The model under review builds one solid part; all positions refer to its coordinate system, in mm. A direction names the side the tool comes from. Coordinates: 2 decimals unless noted, no trailing zeros. Loops run counter-clockwise (first coordinate to the right, second up) from the corner with the lowest first, then second, coordinate; pieces in that order, holes last. Notation, with made-up numbers: (-23.5, 41) - (27.5, 41) arc R7 cw to (27.5, 54) - close; hole circle Ø5 at (50.25, -15.5). An arc over 180 degrees is marked (long way). Answer in a Markdown table with one row per item. Add a question column.
(1) We need section C-C on z = 113.5. Write out the cut boundary in (x, y).
(2) We need section D-D on y = 113. Write out the cut boundary in (x, z).
(3) Mouldability with a two-part tool opening along X and no side actions: class faces 3 (the cylindrical face through (95.38, 30.04, 152.97)), 4 (the flat face through (-95, -29, 310)), 5 (the cylindrical face through (52.684, 82.634, 152.83)) as +X half, -X half, draft (parallel to the pull), parting line (faces both ways), or undercut.
(4) We need section A-A on y = 0. Write out the cut boundary in (x, z).
(5) For P1, Ø4, axis at y = -37, z = 194, coming from the +X side (3 decimals); P2, Ø2, axis at y = 28.5, z = 68, coming from the +X side; P3, Ø5, axis at y = 25.5, z = 44.5, coming from the +X side, all flat-tipped, find the tip position at first contact; note any pin that passes through.
(6) Machinability: for faces 1 (the flat face through (-95, -29, 0)), 2 (the flat face through (-95, 33, 10)), which of the approach directions +Z, -Z, +X, -X, +Y, -Y give a long, thin tool a straight path to every point of the face, cutting with its end or side? Answer none if there is none.
(7) For line 1 along Z through (x, y) = (37, 103.5); line 2 along Y through (x, z) = (0, 138); line 3 along X through (y, z) = (-38, 24), list the stretches that pass through material, from the lowest coordinate up.
from build123d import *

# Parameters (mm, degrees)
SKETCH2_R           = 100
SKETCH2_R_2         = 98
EXTRUDE_THIN1_DEPTH = 310
SKETCH3_R           = 140
SKETCH3_R_2         = 100
BOSS_EXTRUDE1_DEPTH = 10


with BuildPart() as part:
    # Sketch2 → Extrude-Thin1 (new body)
    with BuildSketch(Plane.XY):
        Circle(SKETCH2_R)
        Circle(SKETCH2_R_2, mode=Mode.SUBTRACT)
    extrude(amount=EXTRUDE_THIN1_DEPTH)

    # Sketch3 → Boss-Extrude1 (add)
    with BuildSketch(Plane.XY.offset(310)):
        Circle(SKETCH3_R)
        Circle(SKETCH3_R_2, mode=Mode.SUBTRACT)
    boss_extrude1 = extrude(amount=-BOSS_EXTRUDE1_DEPTH)

    # Mirror1: Boss-Extrude1 across plane
    add(boss_extrude1.mirror(Plane.XY.offset(155)))


solid = part.part
Outcome:
| question | item | result |
|---|---|---|
| 1 | outline | circle Ø200 at (0, 0); hole circle Ø196 at (0, 0) |
| 2 | outline | (-82.65, 0) - (82.65, 0) - (82.65, 10) - (-82.65, 10) - close; (-82.65, 300) - (82.65, 300) - (82.65, 310) - (-82.65, 310) - close |
| 3 | face 3 | parting line |
| 3 | face 4 | draft |
| 3 | face 5 | undercut |
| 4 | outline | (-140, 0) - (-98, 0) - (-98, 310) - (-140, 310) - (-140, 300) - (-100, 300) - (-100, 10) - (-140, 10) - close; (98, 0) - (140, 0) - (140, 10) - (100, 10) - (100, 300) - (140, 300) - (140, 310) - (98, 310) - close |
| 5 | P1 | x = 93.675 |
| 5 | P2 | x = 96.14 |
| 5 | P3 | x = 97.32 |
| 6 | face 1 | -Z, +X, -X, +Y, -Y |
| 6 | face 2 | none |
| 7 | line 1 | 0 to 10, 300 to 310 |
| 7 | line 2 | -100 to -98, 98 to 100 |
| 7 | line 3 | -92.5 to -90.33, 90.33 to 92.5 |
